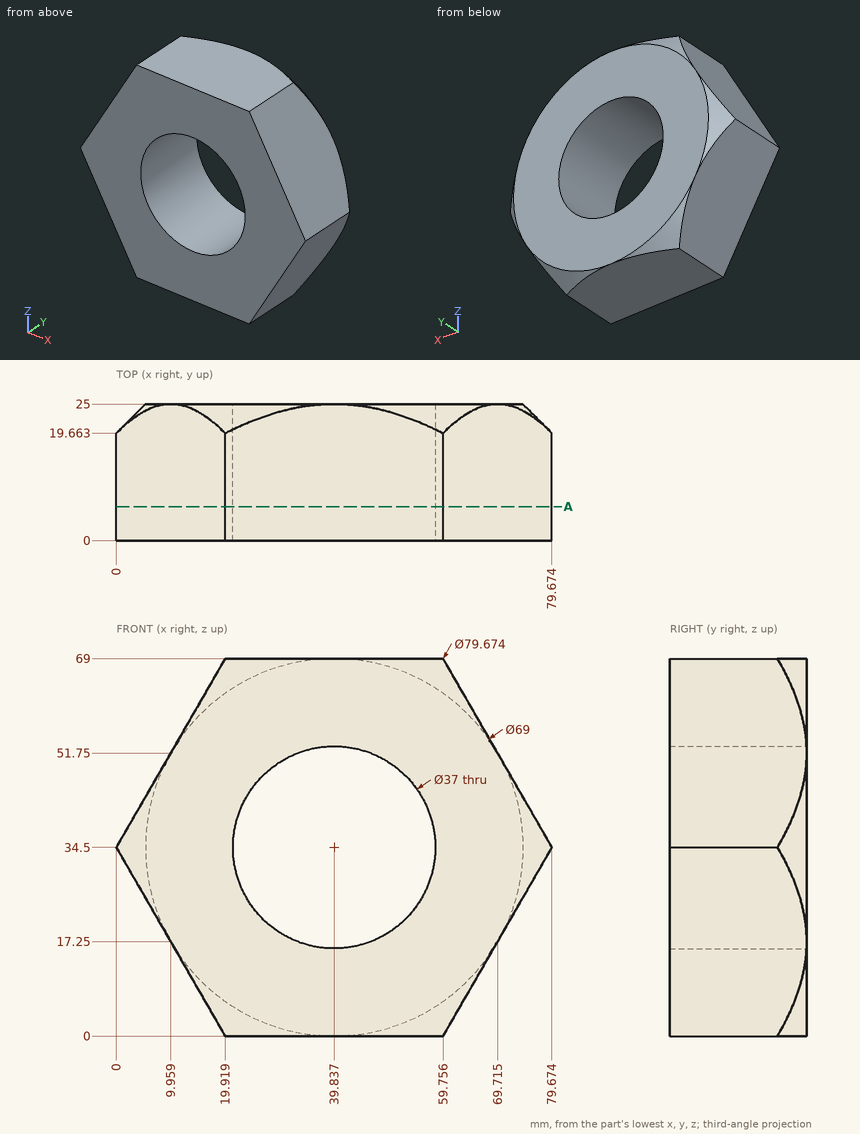
Design review of the part shown in the three views and the two pictorial views. Dimensions are in mm from the part's minimum x, y and z. Give positions to 0.01 mm unless a question says otherwise; leave off trailing zeros. Write each loop counter-clockwise with the first axis right and the second up, starting at its lowest first coordinate (ties: lowest second). Pieces come first, ordered by that corner, then holes. Notation, with made-up numbers: M -16,85.5 L -8,85.5 A20 ccw -8,124.5 Z; hole C 3.5,62.25 d2. An arc over 180 degrees is marked long. Return JSON: item names as keys, results as strings. Group by question number.
Item 1: Clearance check with flat-ended pins moving along their axes: pin 1 Ø2 at (y, z) = (8.5, 10) entering from +X; pin 2 Ø6 at (y, z) = (11, 55.5) entering from -X; pin 3 Ø3 at (x, y) = (19, 19) entering from +Z. State where each tip first meets the part, or that it passes through.
Item 2: Take a section at A-A (y = 6.25). Give the boundary of the cut face in (x, z) (1 decimal).
Item 3: Wall thickness on line 1 along X through (y, z) = (8.25, 34.5) (1 decimal); line 2 along Z through (x, y) = (69, 10.25) (1 decimal); line 3 along Z through (x, y) = (31, 14.75): over which ranges is each line inside the solid? List them lowest first.
Return value:
{
 "1": {"pin 1": "stops at x = 66.11", "pin 2": "stops at x = 10.39", "pin 3": "stops at z = 69"},
 "2": {"outline": "M 0,34.5 L 19.9,0 L 59.8,0 L 79.7,34.5 L 59.8,69 L 19.9,69 Z; hole C 39.8,34.5 d37"},
 "3": {"line 1": "x = 0 to 21.3, 58.3 to 79.7", "line 2": "z = 16 to 53", "line 3": "z = 0 to 18.25, 50.75 to 69"}
}
